from build123d import *

# Parameters (mm, degrees)
SKETCH1_R           = 11
SKETCH1_R_2         = 5.75
BOSS_EXTRUDE1_DEPTH = 9
SKETCH2_R           = 11
CUT_EXTRUDE1_DEPTH  = 8
SKETCH8_R           = 1.25
CUT_EXTRUDE2_DEPTH  = 10


with BuildPart() as part:
    # Sketch1 → Boss-Extrude1 (new body)
    with BuildSketch(Plane(origin=(0, 0, 0), x_dir=(1, 0, 0), z_dir=(0, 1, 0))):
        with BuildLine():
            Line((30, 0), (30, 20))
            ThreePointArc((30, 20), (15, 35), (0, 20))
            Line((0, 20), (0, 0))
            Line((0, 0), (30, 0))
        make_face()
        with Locations((15, 20)):
            Circle(SKETCH1_R, mode=Mode.SUBTRACT)
        with Locations((15, 20)):
            Circle(SKETCH1_R)
        with Locations((15, 20)):
            Circle(SKETCH1_R_2, mode=Mode.SUBTRACT)
    extrude(amount=BOSS_EXTRUDE1_DEPTH)

    # Sketch2 → Cut-Extrude1 (cut)
    with BuildSketch(Plane(origin=(0, 9, 0), x_dir=(1, 0, 0), z_dir=(0, 1, 0))):
        with Locations((15, 20)):
            Circle(SKETCH2_R)
    extrude(amount=-CUT_EXTRUDE1_DEPTH, mode=Mode.SUBTRACT)

    # Sketch8 → Cut-Extrude2 (cut)
    with BuildSketch(Plane.XY):
        with Locations((25, 4.5)):
            Circle(SKETCH8_R)
        with Locations((5, 4.5)):
            Circle(SKETCH8_R)
    extrude(amount=-CUT_EXTRUDE2_DEPTH, mode=Mode.SUBTRACT)


solid = part.part
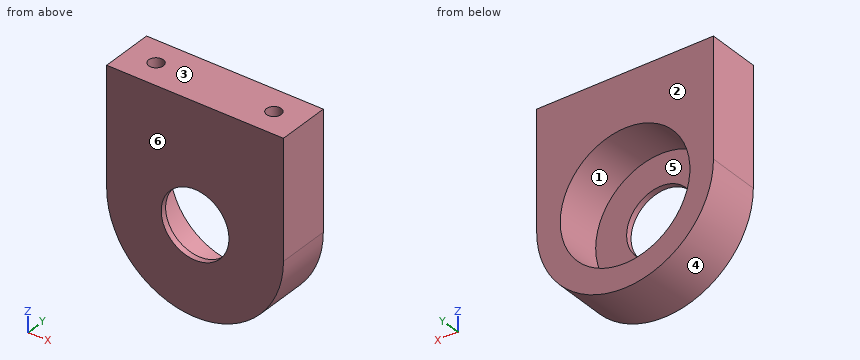
Check sheet for the modelled part. Datum: model origin and axes. Units: mm. Face numbers are marked on the shaded views. A direction names the side the tool comes from. Give positions to 0.01 mm unless a question says otherwise; leave off trailing zeros. Loops run counter-clockwise (first coordinate to the right, second up) from the corner with the lowest first, then second, coordinate; pieces in that order, holes last. Notation, with made-up numbers: M -11.75,29 L 39.25,29 A25 ccw 39.25,51 Z; hole C -9,69 d10. An arc over 180 degrees is marked long. Use a Markdown table: item, result. Add a question column.
Q1. Go/stop test with flat-tipped pins: pin 1 (1.5 mm diameter, centred on x = 5, y = 4.5, fed in from -Z); pin 2 (10 mm diameter, centred on x = 11.5, z = -15.5, fed in from -Y); pin 3 (2 mm diameter, centred on x = 25, y = 4.5, fed in from +Z); pin 4 (2 mm diameter, centred on x = 8, z = -15.5, fed in from +Y). Record where each tip stops, or that it passes through.
Q2. Scan lines: line 1 along Z through (x, y) = (15, 0.35); line 2 along Z through (x, y) = (15, 4.25); line 3 along X through (y, z) = (0.55, -20). Record each from-to range of solid material in increasing order. Write a range as [from, to].
Q3. Sectioned sample at B-B, the plane x = 15. Record the cut outline in (y, z), then the cut area to 4 significant figures.
Q4. Sectioned sample at C-C, the plane z = -4. Record the cut outline in (x, y).
Q5. Sectioned sample at A-A, the plane y = 5.25. Record the cut outline in (x, z).
Q6. Tool access check on the marked faces 5 and 6. Record the directions out of +Z, -Z, +X, -X, +Y, -Y that give a thin tool (end or side, any length) a straight path to the whole face; none if there is none.
Q7. Sectioned sample at D-D, the plane z = -15.5. Record the cut outline in (x, y).
Q8. Mould release check, pull along Z, two halves, no side actions. Record for the marked faces 1, 2, 3 and 4: pulls with the +Z half, pulls with the -Z half, needs draft (parallel to the pull), parting line crosses it, or undercut.
Verdict:
| question | item | result |
|---|---|---|
| 1 | pin 1 | z = -31.81 |
| 1 | pin 2 | y = 0 |
| 1 | pin 3 | z = -10 |
| 1 | pin 4 | y = 1 |
| 2 | line 1 | [-35, -25.75], [-14.25, 0] |
| 2 | line 2 | [-35, -31], [-9, 0] |
| 2 | line 3 | [0, 9.25], [20.75, 30] |
| 3 | outline | M 0,-35 L 9,-35 L 9,-31 L 1,-31 L 1,-25.75 L 0,-25.75 Z; M 0,-14.25 L 1,-14.25 L 1,-9 L 9,-9 L 9,0 L 0,0 Z |
| 3 | area | 127.5 mm^2 |
| 4 | outline | M 0,0 L 30,0 L 30,9 L 0,9 Z; hole C 5,4.5 d2.5; hole C 25,4.5 d2.5 |
| 5 | outline | M 0,-20 A15 ccw 30,-20 L 30,0 L 26,0 L 26,-10 L 24,-10 L 24,0 L 6,0 L 6,-10 L 4,-10 L 4,0 L 0,0 Z; hole C 15,-20 d22 |
| 6 | face 5 | +Y |
| 6 | face 6 | +Z, -Z, +X, -X, -Y |
| 7 | outline | M 0,0 L 11.42,0 L 11.42,1 L 4.96,1 L 4.96,9 L 0,9 Z; M 18.58,0 L 30,0 L 30,9 L 25.04,9 L 25.04,1 L 18.58,1 Z |
| 8 | face 1 | undercut |
| 8 | face 2 | needs draft |
| 8 | face 3 | pulls with the +Z half |
| 8 | face 4 | pulls with the -Z half |
